Here's the drawing with two shaded views (mm, measured from the low corner). I have some questions. Coordinates: 2 decimals unless noted, no trailing zeros. Write each loop counter-clockwise with the first axis right and the second up, starting at its lowest first coordinate (ties: lowest second). Pieces come first, ordered by that corner, then holes.
Item 1: I want a section at C-C on x = 100. Please give me the cut outline in (y, z), then the cut area to 3 significant figures.
Item 2: I want a section at D-D on y = 73. Please give me the cut outline in (x, z).
Item 3: I want a section at A-A on y = 123. Please give me the cut outline in (x, z), then the cut area to 3 significant figures.
Item 4: If I drill on probe 1 along X at (y, z) = (146, 2.25); probe 2 along Y at (x, z) = (133, 5.75); probe 3 along X at (y, z) = (55.5, 2.25), over which ranges is the centre line in solid material (lowest first)?
Item 5: For P1, Ø2.5, axis at x = 27, y = 146, coming from the -Z side, with a flat end and sliding along its axis, tell me the tip position at first contact or that it passes through.
Item 6: I want a section at B-B on x = 156. Please give me the cut outline in (y, z).
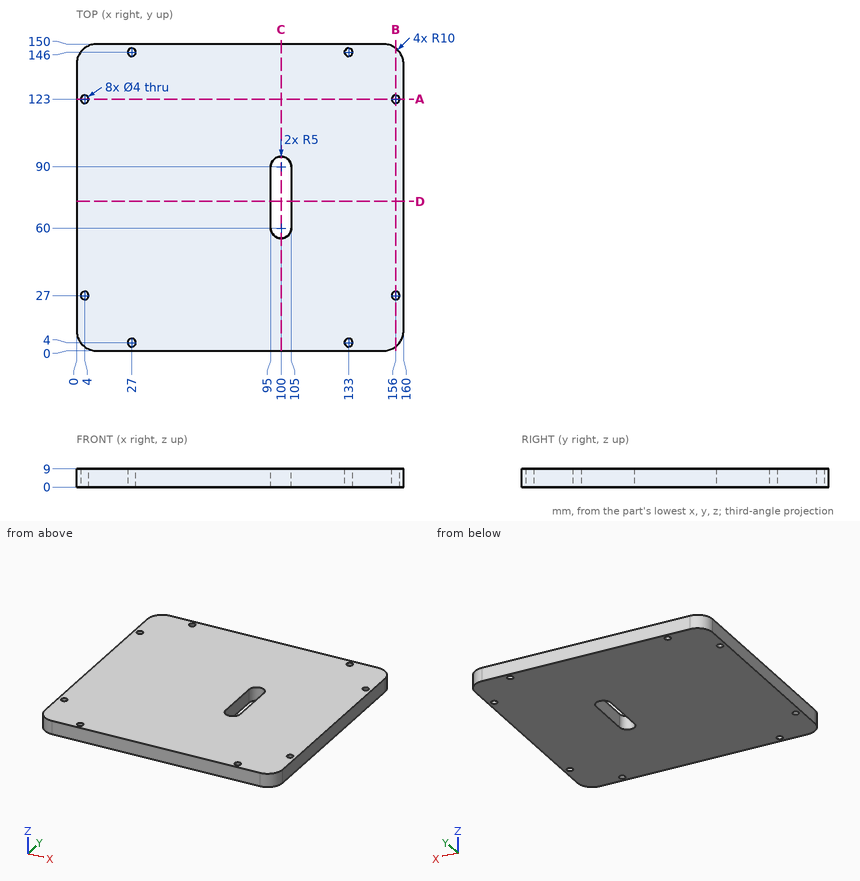
Response values:
1. outline: (0, 0) - (55, 0) - (55, 9) - (0, 9) - close; (95, 0) - (150, 0) - (150, 9) - (95, 9) - close
1. area: 990 mm2
2. outline: (0, 0) - (95, 0) - (95, 9) - (0, 9) - close; (105, 0) - (160, 0) - (160, 9) - (105, 9) - close
3. outline: (0, 0) - (2, 0) - (2, 9) - (0, 9) - close; (6, 0) - (154, 0) - (154, 9) - (6, 9) - close; (158, 0) - (160, 0) - (160, 9) - (158, 9) - close
3. area: 1,370 mm2
4. probe 1: x = 2 to 25, 29 to 131, 135 to 158
4. probe 2: y = 0 to 2, 6 to 144, 148 to 150
4. probe 3: x = 0 to 97.82, 102.18 to 160
5. P1: passes through
6. outline: (2, 0) - (25, 0) - (25, 9) - (2, 9) - close; (29, 0) - (121, 0) - (121, 9) - (29, 9) - close; (125, 0) - (148, 0) - (148, 9) - (125, 9) - close
